Can you work these out from the model? Positions are in its coordinate system, mm. Face numbers are marked on the shaded views. A direction names the side the tool comes from. Round coordinates to 2 decimals unless told otherwise and drop trailing zeros. Loops run counter-clockwise (first coordinate to the right, second up) from the corner with the lowest first, then second, coordinate; pieces in that order, holes last.
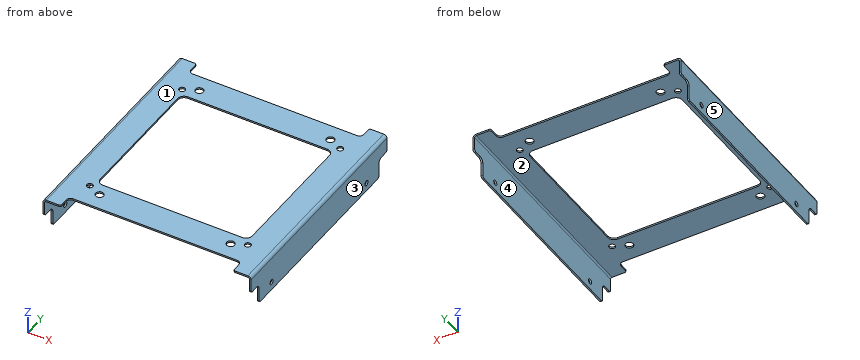
from build123d import *

# Parameters (mm, degrees)
BASE_FLANGE1_DEPTH               = 0.8
EDGE_FLANGE1_STRIP_W             = 4.6732
EDGE_FLANGE1_STRIP_H             = 0.8
EDGE_FLANGE1_STRIP_CUT_DEPTH     = 109
EDGE_FLANGE1_DEPTH               = 109
EDGE_FLANGE2_STRIP_W             = 4.6732
EDGE_FLANGE2_STRIP_H             = 0.8
EDGE_FLANGE2_STRIP_CUT_DEPTH     = 109
EDGE_FLANGE2_DEPTH               = 109
MAIN_START                       = 49.2
MAIN_U_CONNECTORS_OUTLINE_R      = 1.25
MAIN_U_CONNECTORS_DEPTH          = 0.8
SOLAR_START                      = 49.2
SOLAR_PANEL_CONNECTORS_OUTLINE_R = 1.9
SOLAR_PANEL_CONNECTORS_DEPTH     = 0.8
CUT_EXTRUDE2_DEPTH               = 0.8
CUT_EXTRUDE3_DEPTH               = 10
SKETCH21_R                       = 1.45
CUT_EXTRUDE4_DEPTH               = 10
FILLET1_R                        = 1


# Read off the part's stored shape, not the designer's step: Main U Connectors, Solar Panel Connectors 
# Sheet-metal steps are written as plain solids
with BuildPart() as part:
    # Sketch1 → Base-Flange1 (new body)
    with BuildSketch(Plane.XY.offset(50)):
        with BuildLine():
            Line((-39.5, 48), (39.5, 48))
            ThreePointArc((39.5, 48), (40.914213562, 48.585786438), (41.5, 50))
            Line((41.5, 50), (41.5, 54.5))
            Line((41.5, 54.5), (50, 54.5))
            Line((50, 54.5), (50, 48))
            Line((50, 48), (50, -48))
            Line((50, -48), (50, -54.5))
            Line((50, -54.5), (41.5, -54.5))
            Line((41.5, -54.5), (41.5, -50))
            ThreePointArc((41.5, -50), (40.914213562, -48.585786438), (39.5, -48))
            Line((39.5, -48), (-39.5, -48))
            ThreePointArc((-39.5, -48), (-40.914213562, -48.585786438), (-41.5, -50))
            Line((-41.5, -50), (-41.5, -54.5))
            Line((-41.5, -54.5), (-50, -54.5))
            Line((-50, -54.5), (-50, -48))
            Line((-50, -48), (-50, 48))
            Line((-50, 48), (-50, 54.5))
            Line((-50, 54.5), (-41.5, 54.5))
            Line((-41.5, 54.5), (-41.5, 50))
            ThreePointArc((-41.5, 50), (-40.914213562, 48.585786438), (-39.5, 48))
        make_face()
    extrude(amount=-BASE_FLANGE1_DEPTH)

    # Edge-Flange1 strip (across the edge) → Edge-Flange1 strip cut (cut)
    with BuildSketch(Plane(origin=(50, 54.5, 49.2), x_dir=(-1, 0, 0), z_dir=(0, -1, 0))):
        with Locations((-0.8, -0.4)):
            Rectangle(EDGE_FLANGE1_STRIP_W, EDGE_FLANGE1_STRIP_H)
    extrude(amount=EDGE_FLANGE1_STRIP_CUT_DEPTH, mode=Mode.SUBTRACT)

    # Edge-Flange1 section (across the edge) → Edge-Flange1 (add)
    with BuildSketch(Plane(origin=(50, 54.5, 49.2), x_dir=(-1, 0, 0), z_dir=(0, -1, 0))):
        with BuildLine():
            Line((0, 0.7366), (0, 17.2))
            Line((0, 17.2), (0.8, 17.2))
            Line((0.8, 17.2), (0.8, 0.7366))
            ThreePointArc((0.8, 0.7366), (1.015745145, 0.215745145), (1.5366, 0))
            Line((1.5366, 0), (1.5366, -0.8))
            ThreePointArc((1.5366, -0.8), (0.45005972, -0.34994028), (0, 0.7366))
        make_face()
    extrude(amount=EDGE_FLANGE1_DEPTH)

    # Edge-Flange2 strip (across the edge) → Edge-Flange2 strip cut (cut)
    with BuildSketch(Plane(origin=(-50, -54.5, 49.2), x_dir=(1, 0, 0), z_dir=(0, 1, 0))):
        with Locations((-0.8, -0.4)):
            Rectangle(EDGE_FLANGE2_STRIP_W, EDGE_FLANGE2_STRIP_H)
    extrude(amount=EDGE_FLANGE2_STRIP_CUT_DEPTH, mode=Mode.SUBTRACT)

    # Edge-Flange2 section (across the edge) → Edge-Flange2 (add)
    with BuildSketch(Plane(origin=(-50, -54.5, 49.2), x_dir=(1, 0, 0), z_dir=(0, 1, 0))):
        with BuildLine():
            Line((0, 0.7366), (0, 17.2))
            Line((0, 17.2), (0.8, 17.2))
            Line((0.8, 17.2), (0.8, 0.7366))
            ThreePointArc((0.8, 0.7366), (1.015745145, 0.215745145), (1.5366, 0))
            Line((1.5366, 0), (1.5366, -0.8))
            ThreePointArc((1.5366, -0.8), (0.45005972, -0.34994028), (0, 0.7366))
        make_face()
    extrude(amount=EDGE_FLANGE2_DEPTH)

    # Main U Connectors outline → Main U Connectors (cut)
    with BuildSketch(Plane.YZ.offset(MAIN_START)):
        with Locations((-38, 36)):
            Circle(MAIN_U_CONNECTORS_OUTLINE_R)
        with Locations((38, 36)):
            Circle(MAIN_U_CONNECTORS_OUTLINE_R)
    main_u_connectors = extrude(amount=MAIN_U_CONNECTORS_DEPTH, mode=Mode.SUBTRACT)

    # Solar Panel Connectors outline → Solar Panel Connectors (cut)
    with BuildSketch(Plane.XY.offset(SOLAR_START)):
        with Locations((-31.5, 40)):
            Circle(SOLAR_PANEL_CONNECTORS_OUTLINE_R)
        with Locations((31.5, 40)):
            Circle(SOLAR_PANEL_CONNECTORS_OUTLINE_R)
        with Locations((31.5, -40)):
            Circle(SOLAR_PANEL_CONNECTORS_OUTLINE_R)
        with Locations((-31.5, -40)):
            Circle(SOLAR_PANEL_CONNECTORS_OUTLINE_R)
    extrude(amount=SOLAR_PANEL_CONNECTORS_DEPTH, mode=Mode.SUBTRACT)

    # Sketch18 → Cut-Extrude2 (cut)
    with BuildSketch(Plane.XY.offset(50)):
        with BuildLine():
            Line((-33.5, -34), (33.5, -34))
            ThreePointArc((33.5, -34), (35.621320344, -33.121320344), (36.5, -31))
            Line((36.5, -31), (36.5, 31))
            ThreePointArc((36.5, 31), (35.621320344, 33.121320344), (33.5, 34))
            Line((33.5, 34), (-33.5, 34))
            ThreePointArc((-33.5, 34), (-35.621320344, 33.121320344), (-36.5, 31))
            Line((-36.5, 31), (-36.5, -31))
            ThreePointArc((-36.5, -31), (-35.621320344, -33.121320344), (-33.5, -34))
        make_face()
    extrude(amount=-CUT_EXTRUDE2_DEPTH, mode=Mode.SUBTRACT)

    # Sketch19 → Cut-Extrude3 (cut)
    with BuildSketch(Plane(origin=(50, 0, 0), x_dir=(0, 0, -1), z_dir=(1, 0, 0))):
        with BuildLine():
            Line((-32, 54.5), (-41.5, 54.5))
            Line((-41.5, 54.5), (-41.5, 50))
            ThreePointArc((-41.5, 50), (-40.914213562, 48.585786438), (-39.5, 48))
            Line((-39.5, 48), (-32, 48))
            Line((-32, 48), (-32, 54.5))
        make_face()
        with BuildLine():
            Line((-41.5, -54.5), (-41.5, -50))
            ThreePointArc((-41.5, -50), (-40.914213562, -48.585786438), (-39.5, -48))
            Line((-39.5, -48), (-32, -48))
            Line((-32, -48), (-32, -54.5))
            Line((-32, -54.5), (-41.5, -54.5))
        make_face()
    cut_extrude3 = extrude(amount=-CUT_EXTRUDE3_DEPTH, mode=Mode.SUBTRACT)

    # Mirror1: Main U Connectors, Cut-Extrude3 across plane
    add(main_u_connectors.mirror(Plane(origin=(0, 0, 0), x_dir=(0, 0, 1), z_dir=(1, 0, 0))), mode=Mode.SUBTRACT)
    add(cut_extrude3.mirror(Plane(origin=(0, 0, 0), x_dir=(0, 0, 1), z_dir=(1, 0, 0))), mode=Mode.SUBTRACT)

    # Sketch21 → Cut-Extrude4 (cut)
    with BuildSketch(Plane.XY.offset(50)):
        with Locations((-38, 37)):
            Circle(SKETCH21_R)
        with Locations((38, 37)):
            Circle(SKETCH21_R)
        with Locations((38, -37)):
            Circle(SKETCH21_R)
        with Locations((-38, -37)):
            Circle(SKETCH21_R)
    extrude(amount=-CUT_EXTRUDE4_DEPTH, mode=Mode.SUBTRACT)

    # Fillet1
    fillet1_edges = [part.edges().sort_by_distance(p)[0] for p in [
        (49.6, 48, 32),
        (49.6, 54.5, 41.5),
        (49.6, -48, 32),
        (49.6, -54.5, 41.5),
        (-49.6, 48, 32),
        (-49.6, 54.5, 41.5),
        (-49.6, -54.5, 41.5),
        (-49.6, -48, 32),
        (-41.5, 54.5, 49.6),
        (41.5, 54.5, 49.6),
        (41.5, -54.5, 49.6),
        (-41.5, -54.5, 49.6),
    ]]
    fillet(fillet1_edges, radius=FILLET1_R)


solid = part.part
(1) If we mould it in two halves opening along X, with no side actions, what happens to the marked faces 1, 2 and 3? For each: released by +X, released by -X, zero draft, split by the parting line, or undercut.
Worked answers:
face 1: zero draft
face 2: undercut
face 3: released by +X
(2) If we section it at A-A, the plane y = 9: List the corners of the cut face in (x, z) for me.
Worked answers:
outline: (-50, 32) - (-49.2, 32) - (-49.2, 48.46) arc R0.74 cw to (-48.46, 49.2) - (-36.5, 49.2) - (-36.5, 50) - (-48.46, 50) arc R1.54 ccw to (-50, 48.46) - close; (36.5, 49.2) - (48.46, 49.2) arc R0.74 cw to (49.2, 48.46) - (49.2, 32) - (50, 32) - (50, 48.46) arc R1.54 ccw to (48.46, 50) - (36.5, 50) - close
(3) If I drill on line 1 (Y direction, x = 31.5, z = 49.8); line 2 (Y direction, x = 38, z = 49.6); line 3 (X direction, y = -47, z = 45.5), over which ranges is the centre line in solid material (lowest first)?
Worked answers:
line 1: y = -48 to -41.9, -38.1 to -34, 34 to 38.1, 41.9 to 48
line 2: y = -48 to -38.45, -35.55 to 35.55, 38.45 to 48
line 3: x = -50 to -49.2, 49.2 to 50
(4) If we section it at C-C, the plane x = 38: List the corners of the cut face in (y, z) for me.
Worked answers:
outline: (-48, 49.2) - (-38.45, 49.2) - (-38.45, 50) - (-48, 50) - close; (-35.55, 49.2) - (35.55, 49.2) - (35.55, 50) - (-35.55, 50) - close; (38.45, 49.2) - (48, 49.2) - (48, 50) - (38.45, 50) - close
(5) If we section it at D-D, the plane x = 22: List the corners of the cut face in (y, z) for me.
Worked answers:
outline: (-48, 49.2) - (-34, 49.2) - (-34, 50) - (-48, 50) - close; (34, 49.2) - (48, 49.2) - (48, 50) - (34, 50) - close
(6) If we section it at B-B, the plane z = 36: List the corners of the cut face in (x, y) for me.
Worked answers:
outline: (-50, -48) - (-49.2, -48) - (-49.2, -39.25) - (-50, -39.25) - close; (-50, -36.75) - (-49.2, -36.75) - (-49.2, 36.75) - (-50, 36.75) - close; (-50, 39.25) - (-49.2, 39.25) - (-49.2, 48) - (-50, 48) - close; (49.2, -48) - (50, -48) - (50, -39.25) - (49.2, -39.25) - close; (49.2, -36.75) - (50, -36.75) - (50, 36.75) - (49.2, 36.75) - close; (49.2, 39.25) - (50, 39.25) - (50, 48) - (49.2, 48) - close
(7) Will these pins go through, and if not, where does the flat tip stop? P1, Ø0.9, axis at x = -49.5, y = -51, coming from the -Z side; P2, Ø0.6, axis at x = 50, z = 36.5, coming from the +Y side; P3, Ø4.5, axis at x = -38, y = 37, coming from the -Z side.
Worked answers:
P1: stops at z = 41.5
P2: stops at y = 48
P3: stops at z = 49.2
(8) For the marked faces 4 and 5, which set-ups out of +Z, -Z, +X, -X, +Y, -Y let a thin tool reach every point of the face, with its end or its side?
Worked answers:
face 4: -Z, +Y, -Y
face 5: +Z, -Z, -X, +Y, -Y
